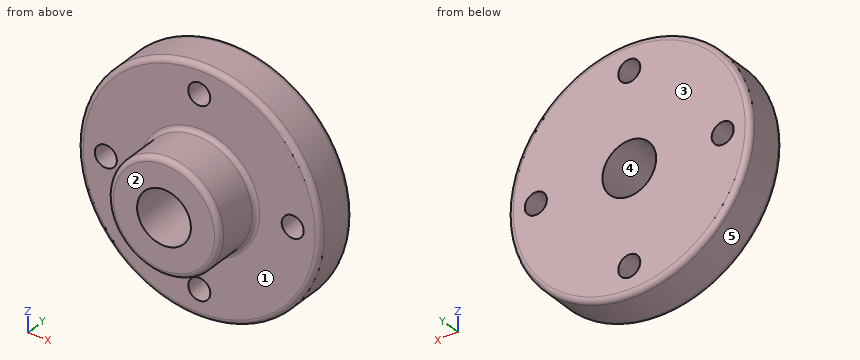
```python
from build123d import *

# Parameters (mm, degrees)
F0_R            = 69.85
F1_DEPTH        = 25.4
F2_R            = 19.05
F2_R_2          = 6.35
F3_DEPTH        = 25.401
F3_COPIES_COUNT = 4
F6_R            = 3.048
F7_R            = 3.048
F8_R            = 2.54


# Not quite as in the source:
# - a pattern or mirror of a feature is missing from the dataset's text; its kind, count and spacing are read off the source's solid


with BuildPart() as f1:
    # F0 (on Front) → F1 (new body)
    with BuildSketch(Plane.XZ):
        Circle(F0_R)
    extrude(amount=F1_DEPTH)

    # F2 (on Front) → F3 (cut, through all)
    with BuildSketch(Plane.XZ):
        Circle(F2_R)
        with Locations((0, 53.848)):
            Circle(F2_R_2)
    f3 = extrude(amount=F3_DEPTH, mode=Mode.SUBTRACT)

    # F3_copies: F3 ×4 about axis
    f3_copies_axis = Axis((0, 0, 0), (0, 1, 0))
    for i in range(1, F3_COPIES_COUNT):
        add(f3.rotate(f3_copies_axis, i * 360 / F3_COPIES_COUNT), mode=Mode.SUBTRACT)

    # F4 (on Right) → F5 (revolve)
    with BuildSketch(Plane.YZ):
        with BuildLine():
            Line((-53.848, 15.4953468409), (0, 15.4953468409))
            Line((0, 15.4953468409), (0, 32.2310491102))
            Line((0, 32.2310491102), (-25.3001134843, 32.2310491102))
            Line((-25.3001134843, 32.2310491102), (-50.8, 32.2310491102))
            ThreePointArc((-50.8, 32.2310491102), (-52.9552614691, 31.3383105793), (-53.848, 29.1830491102))
            Line((-53.848, 29.1830491102), (-53.848, 15.4953468409))
        make_face()
    revolve(axis=Axis((0, -22.6452342175, 0), (0, -1, 0)))

    # F6
    f6_edges = [f1.edges().sort_by_distance(p)[0] for p in [
        (-69.85, -25.4, 0),
    ]]
    fillet(f6_edges, radius=F6_R)

    # F7
    f7_edges = [f1.edges().sort_by_distance(p)[0] for p in [
        (-69.85, 0, 0),
    ]]
    fillet(f7_edges, radius=F7_R)

    # F8
    f8_edges = [f1.edges().sort_by_distance(p)[0] for p in [
        (0, -25.4, -32.231049),
    ]]
    fillet(f8_edges, radius=F8_R)


solid = f1.part
```
Verification items for the finished model (mm, model axes). Face numbers are marked on the shaded views. A direction names the side the tool comes from. Coordinates: 2 decimals unless noted, no trailing zeros. Loops run counter-clockwise (first coordinate to the right, second up) from the corner with the lowest first, then second, coordinate; pieces in that order, holes last. Notation, with made-up numbers: (52.25, -23) - (90.25, -23) arc R8 ccw to (90.25, -10) - close; hole circle Ø2 at (46.25, 66). An arc over 180 degrees is marked (long way). Answer as a JSON object with one key per item and string values.
(1) Scan lines: line 1 along Z through (x, y) = (0, -18); line 2 along X through (y, z) = (-43, 0); line 3 along Z through (x, y) = (-4, -19.5). Record each from-to range of solid material in increasing order.
Response:
{"line 1": "z = -69.85 to -60.2, -47.5 to -15.5, 15.5 to 47.5, 60.2 to 69.85", "line 2": "x = -32.23 to -15.5, 15.5 to 32.23", "line 3": "z = -69.74 to -58.78, -48.92 to -14.97, 14.97 to 48.92, 58.78 to 69.74"}
(2) Cross-section at C-C, the plane y = -30.5. Record the boundary of the cut face in (x, z), then the cut area to 3 significant figures.
Response:
{"outline": "circle Ø64.46 at (0, 0); hole circle Ø30.99 at (0, 0)", "area": "2,510 mm²"}
(3) Mould release check, pull along Z, two halves, no side actions. Record for the marked faces 3, 4 and 5: pulls with the +Z half, pulls with the -Z half, needs draft (parallel to the pull), parting line crosses it, or undercut.
Response:
{"face 3": "needs draft", "face 4": "undercut", "face 5": "parting line crosses it"}
(4) Go/stop test with flat-tipped pins: pin 1 Ø12 at (x, y) = (-30.5, -19) entering from -Z; pin 2 Ø6 at (x, z) = (-8.5, 41) entering from -Y; pin 3 Ø2 at (y, z) = (-43, -23) entering from +X; pin 4 Ø11.5 at (x, z) = (-53.848, 0) entering from +Y. Record where each tip stops, or that it passes through.
Response:
{"pin 1": "stops at z = -65.41", "pin 2": "stops at y = -25.4", "pin 3": "stops at x = 23.56", "pin 4": "passes through"}
(5) Access from +Z, -Z, +X, -X, +Y, -Y to the whole of each face (thin tool, end or side, straight path). Record for the marked faces 1 and 2.
Response:
{"face 1": "-Y", "face 2": "+Z, -Z, +X, -X, -Y"}
(6) Cross-section at A-A, the plane x = 0. Record the boundary of the cut face in (y, z).
Response:
{"outline": "(-53.85, -29.18) arc R3.05 ccw to (-50.8, -32.23) - (-27.94, -32.23) arc R2.54 cw to (-25.4, -34.77) - (-25.4, -47.5) - (0, -47.5) - (0, -15.5) - (-53.85, -15.5) - close; (-53.85, 15.5) - (0, 15.5) - (0, 47.5) - (-25.4, 47.5) - (-25.4, 34.77) arc R2.54 cw to (-27.94, 32.23) - (-50.8, 32.23) arc R3.05 ccw to (-53.85, 29.18) - close; (-25.4, -66.8) arc R3.05 ccw to (-22.35, -69.85) - (-3.05, -69.85) arc R3.05 ccw to (0, -66.8) - (0, -60.2) - (-25.4, -60.2) - close; (-25.4, 60.2) - (0, 60.2) - (0, 66.8) arc R3.05 ccw to (-3.05, 69.85) - (-22.35, 69.85) arc R3.05 ccw to (-25.4, 66.8) - close"}
(7) Cross-section at B-B, the plane z = 0. Record the boundary of the cut face in (x, y), then the cut area to 3 significant figures.
Response:
{"outline": "(-69.85, -22.35) arc R3.05 ccw to (-66.8, -25.4) - (-60.2, -25.4) - (-60.2, 0) - (-66.8, 0) arc R3.05 ccw to (-69.85, -3.05) - close; (-47.5, -25.4) - (-34.77, -25.4) arc R2.54 cw to (-32.23, -27.94) - (-32.23, -50.8) arc R3.05 ccw to (-29.18, -53.85) - (-15.5, -53.85) - (-15.5, 0) - (-47.5, 0) - close; (15.5, -53.85) - (29.18, -53.85) arc R3.05 ccw to (32.23, -50.8) - (32.23, -27.94) arc R2.54 cw to (34.77, -25.4) - (47.5, -25.4) - (47.5, 0) - (15.5, 0) - close; (60.2, -25.4) - (66.8, -25.4) arc R3.05 ccw to (69.85, -22.35) - (69.85, -3.05) arc R3.05 ccw to (66.8, 0) - (60.2, 0) - close", "area": "3,060 mm²"}
